Check sheet for the drawn part. Datum: minimum x, y, z corner. Units: mm. A direction names the side the tool comes from. Give positions to 0.01 mm unless a question says otherwise; leave off trailing zeros. Order: outer loops, then holes, each group sorted by start corner. A loop starts at its lowest first (then second) coordinate and runs counter-clockwise, first axis right, second up. Notation, with made-up numbers: (59.5, -37) - (97.5, -37) arc R19 ccw to (97.5, -29) - close; hole circle Ø2 at (5, -21.75). An arc over 180 degrees is marked (long way). Answer as a JSON object with one key per item and string values. Group by question number.
(1) Section check A-A (z = 1). Record the boundary of the cut face in (x, y) (1 decimal), then the cut area to 3 significant figures.
(2) Section check D-D (x = 5). Record the boundary of the cut face in (y, z).
(3) Thickness scan on line 1 (X direction, y = 17, z = 2.85) (1 decimal); line 2 (Y direction, x = 9, z = 1.55) (1 decimal); line 3 (X direction, y = 18, z = 2.8) (1 decimal). Record the ranges inside material, lowest first.
(4) Section check B-B (y = 24.5). Record the boundary of the cut face in (x, z) (1 decimal).
(5) Depth check by flat-ended pin: pin 1 Ø1.5 at (x, z) = (26.5, 1) entering from +Y (1 decimal); pin 2 Ø0.9 at (x, z) = (24, 1) entering from +Y; pin 3 Ø1 at (y, z) = (11, 1) entering from -X (1 decimal). Enter the tip coordinate at first touch or a pass-through.
(6) Access from +Z, -Z, +X, -X, +Y, -Y to the whole of each face (thin tool, end or side, straight path). Record for the marked faces 1 and 2.
(7) Section check C-C (y = 17). Record the boundary of the cut face in (x, z).
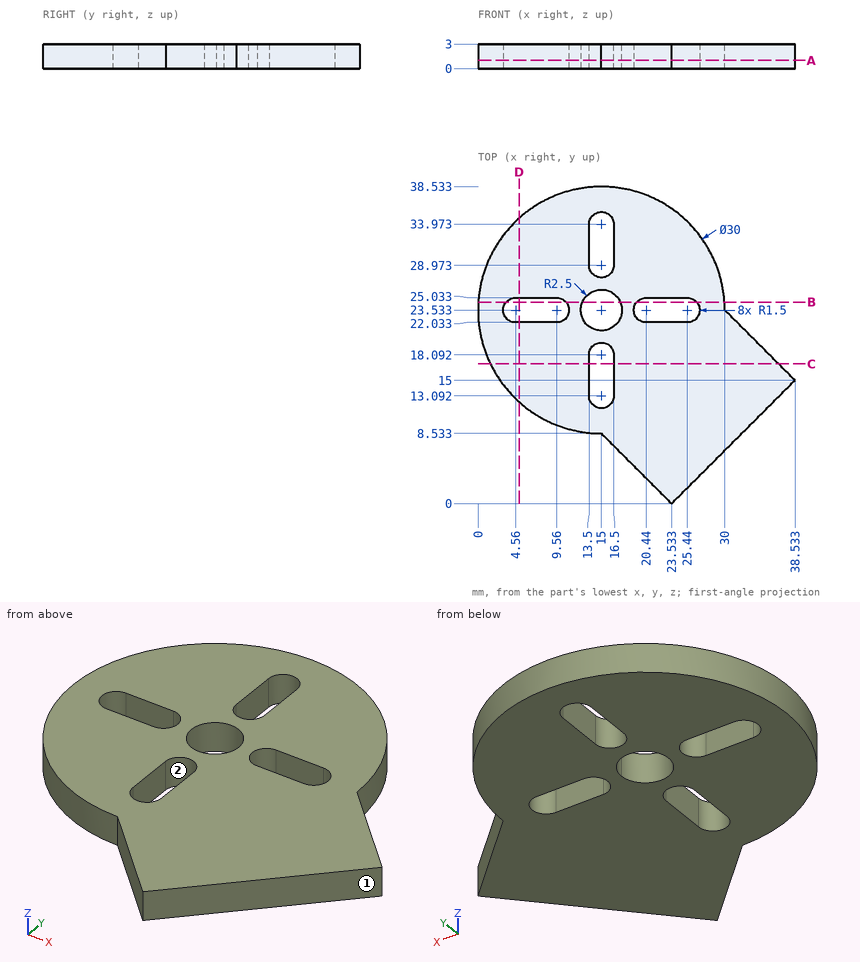
Solutions:
{
 "1": {"outline": "(15, 8.5) - (23.5, 0) - (38.5, 15) - (30, 23.5) arc R15 ccw (long way) to start; hole (4.6, 22) - (9.6, 22) arc R1.5 ccw to (9.6, 25) - (4.6, 25) arc R1.5 ccw to start; hole (13.5, 13.1) arc R1.5 ccw to (16.5, 13.1) - (16.5, 18.1) arc R1.5 ccw to (13.5, 18.1) - close; hole (13.5, 29) arc R1.5 ccw to (16.5, 29) - (16.5, 34) arc R1.5 ccw to (13.5, 34) - close; hole (16.8, 25.3) arc R2.5 ccw (long way) to (17.5, 23.5) arc R2.5 ccw to start; hole (20.4, 22) - (25.4, 22) arc R1.5 ccw to (25.4, 25) - (20.4, 25) arc R1.5 ccw to start", "area": "791 mm2"},
 "2": {"outline": "(12.35, 0) - (22.03, 0) - (22.03, 3) - (12.35, 3) - close; (25.03, 0) - (34.71, 0) - (34.71, 3) - (25.03, 3) - close"},
 "3": {"line 1": "x = 1.5 to 13.5, 16.5 to 36.5", "line 2": "y = 9.8 to 22, 25 to 37.3", "line 3": "x = 1.1 to 13.5, 16.5 to 35.5"},
 "4": {"outline": "(0, 0) - (3.4, 0) - (3.4, 3) - (0, 3) - close; (10.7, 0) - (12.7, 0) - (12.7, 3) - (10.7, 3) - close; (17.3, 0) - (19.3, 0) - (19.3, 3) - (17.3, 3) - close; (26.6, 0) - (30, 0) - (30, 3) - (26.6, 3) - close"},
 "5": {"pin 1": "stops at y = 34", "pin 2": "stops at y = 35.86", "pin 3": "stops at x = 6"},
 "6": {"face 1": "+Z, -Z, +X, -Y", "face 2": "+Z, -Z"},
 "7": {"outline": "(1.5, 0) - (13.5, 0) - (13.5, 3) - (1.5, 3) - close; (16.5, 0) - (36.53, 0) - (36.53, 3) - (16.5, 3) - close"}
}
